```python
from build123d import *

# Parameters (mm, degrees)
ESQUISSE1_W             = 30
ESQUISSE1_H             = 30
BOSS_EXTRU_1_DEPTH      = 11
TROU_TARAUD_M31_D       = 2.5
ENL_V_MAT_EXTRU_1_REACH = 25.896
ESQUISSE6_R             = 10.5
BOSS_EXTRU_2_DEPTH      = 3.5
ESQUISSE7_R             = 8.75
BOSS_EXTRU_3_DEPTH      = 0.5
ESQUISSE8_R             = 2.5
BOSS_EXTRU_4_DEPTH      = 4
ESQUISSE9_R             = 2
BOSS_EXTRU_5_DEPTH      = 20
CHANFREIN1_SIZE         = 3
ENL_V_MAT_EXTRU_2_DEPTH = 3


with BuildPart() as part:
    # Esquisse1 → Boss.-Extru.1 (new body)
    with BuildSketch(Plane.XY):
        Rectangle(ESQUISSE1_W, ESQUISSE1_H)
    extrude(amount=BOSS_EXTRU_1_DEPTH)

    # Trou taraudé M31 (through all)
    with Locations(Plane.XY.offset(11)):
        with Locations((11, -11), (-11, 11)):
            Hole(TROU_TARAUD_M31_D / 2)

    # Esquisse5 → Enlèv. mat.-Extru.1 (cut, up to next)
    with BuildSketch(Plane.XY.offset(11), mode=Mode.PRIVATE) as enl_v_mat_extru_1_sk1:
        with BuildLine():
            Line((12.5, 12.5), (7.5, 12.5))
            ThreePointArc((7.5, 12.5), (6, 11), (7.5, 9.5))
            Line((7.5, 9.5), (12.5, 9.5))
            ThreePointArc((12.5, 9.5), (14, 11), (12.5, 12.5))
        make_face()
    enl_v_mat_extru_1_tool1 = extrude(enl_v_mat_extru_1_sk1.sketch, amount=-ENL_V_MAT_EXTRU_1_REACH, mode=Mode.PRIVATE) & part.part
    # Esquisse5 → Enlèv. mat.-Extru.1 (cut, up to next)
    with BuildSketch(Plane.XY.offset(11), mode=Mode.PRIVATE) as enl_v_mat_extru_1_sk2:
        with BuildLine():
            Line((-7.5, -9.5), (-12.5, -9.5))
            ThreePointArc((-12.5, -9.5), (-14, -11), (-12.5, -12.5))
            Line((-12.5, -12.5), (-7.5, -12.5))
            ThreePointArc((-7.5, -12.5), (-6, -11), (-7.5, -9.5))
        make_face()
    enl_v_mat_extru_1_tool2 = extrude(enl_v_mat_extru_1_sk2.sketch, amount=-ENL_V_MAT_EXTRU_1_REACH, mode=Mode.PRIVATE) & part.part
    add(enl_v_mat_extru_1_tool1.solids().sort_by_distance((10, 11, 11))[0], mode=Mode.SUBTRACT)
    add(enl_v_mat_extru_1_tool2.solids().sort_by_distance((-10, -11, 11))[0], mode=Mode.SUBTRACT)

    # Esquisse6 → Boss.-Extru.2 (add)
    with BuildSketch(Plane.XY.offset(11)):
        Circle(ESQUISSE6_R)
    extrude(amount=BOSS_EXTRU_2_DEPTH)

    # Esquisse7 → Boss.-Extru.3 (add)
    with BuildSketch(Plane.XY.offset(14.5)):
        Circle(ESQUISSE7_R)
    extrude(amount=BOSS_EXTRU_3_DEPTH)

    # Esquisse8 → Boss.-Extru.4 (add)
    with BuildSketch(Plane(origin=(0, -15, 0), x_dir=(-1, 0, 0), z_dir=(0, -1, 0))):
        with Locations(Location((0, -5.5, 0), (0, 0, 270))):
            Circle(ESQUISSE8_R)
    extrude(amount=BOSS_EXTRU_4_DEPTH)

    # Esquisse9 → Boss.-Extru.5 (add)
    with BuildSketch(Plane(origin=(0, -19, 0), x_dir=(-1, 0, 0), z_dir=(0, -1, 0))):
        with Locations(Location((0, -5.5, 0), (0, 0, 90))):
            Circle(ESQUISSE9_R)
    extrude(amount=BOSS_EXTRU_5_DEPTH)

    # Chanfrein1
    chanfrein1_edges = [part.edges().sort_by_distance(p)[0] for p in [
        (-15, 15, 5.5),
        (15, 15, 5.5),
        (15, -15, 5.5),
        (-15, -15, 5.5),
    ]]
    chamfer(chanfrein1_edges, length=CHANFREIN1_SIZE)

    # Esquisse10 → Enlèv. mat.-Extru.2 (cut)
    with BuildSketch(Plane(origin=(0, 0, 0), x_dir=(-1, 0, 0), z_dir=(0, 0, -1))):
        with BuildLine():
            Line((-7.5, 8), (-12.5, 8))
            Line((-12.5, 8), (-12.5, -7.964466094))
            Line((-12.5, -7.964466094), (-10.964466094, -7.964466094))
            ThreePointArc((-10.964466094, -7.964466094), (-8.843145751, -8.843145751), (-7.964466094, -10.964466094))
            Line((-7.964466094, -10.964466094), (-7.964466094, -12.5))
            Line((-7.964466094, -12.5), (4.5, -12.5))
            Line((4.5, -12.5), (4.5, -11))
            ThreePointArc((4.5, -11), (5.378679656, -8.878679656), (7.5, -8))
            Line((7.5, -8), (12.5, -8))
            Line((12.5, -8), (12.5, 8))
            Line((12.5, 8), (11, 8))
            ThreePointArc((11, 8), (8.878679656, 8.878679656), (8, 11))
            Line((8, 11), (8, 12.5))
            Line((8, 12.5), (-4.5, 12.5))
            Line((-4.5, 12.5), (-4.5, 11))
            ThreePointArc((-4.5, 11), (-5.378679656, 8.878679656), (-7.5, 8))
        make_face()
    extrude(amount=-ENL_V_MAT_EXTRU_2_DEPTH, mode=Mode.SUBTRACT)


solid = part.part
```
The listing builds one solid part. Answer for the finished solid, in the listing's coordinates (mm). A direction names the side the tool comes from. Give positions to 0.01 mm unless a question says otherwise; leave off trailing zeros. Order: outer loops, then holes, each group sorted by start corner. A loop starts at its lowest first (then second) coordinate and runs counter-clockwise, first axis right, second up. Notation, with made-up numbers: (46, -38.75) - (51, -38.75) arc R14 cw to (51, -31.75) - close; hole circle Ø11 at (-13.5, 71.5). An arc over 180 degrees is marked (long way). Use one line per item in the form item = value. Start each with the question number.
(1) A cutting plane is placed at D-D, the plane z = 5.5. Write down the section's boundary in (x, y).
(2) A cutting plane is placed at B-B, the plane y = 0. Write down the section's boundary in (x, z).
(3) A cutting plane is placed at C-C, the plane x = 0. Write down the section's boundary in (y, z).
(4) Consider line 1 (Y direction, x = -11, z = 7); line 2 (Y direction, x = 11, z = 7.5); line 3 (Y direction, x = 8.5, z = 10). Determine where each line is inside the solid, lowest interval first. Write a range as from..to.
(5) Flat-ended cylindrical pins translate along their axes: pin 1 Ø1 at (x, y) = (3, -1.5) entering from -Z; pin 2 Ø2.5 at (x, z) = (10, 1) entering from -Y; pin 3 Ø6 at (y, z) = (-28.5, 8.5) entering from +X. Find the tip coordinate at first contact, or state that the pin passes through.
(6) A cutting plane is placed at A-A, the plane z = 9.75. Write down the section's boundary in (x, y), then the cut area to 3 significant figures.
(7) The mould has two halves that part along X. Classify faces 1 (the flat face through (-15, 0, 5)), 2 (the flat face through (-4, 8, 14.5)), 3 (the flat face through (-10, -12.5, 6)), 4 (the cylindrical face through (11.921, -10.155, 5.423)): released by +X, released by -X, zero draft, split by the parting line, or undercut.
(8) For faces 5 (the cylindrical face through (-14, -11, 6)), 6 (the cylindrical face through (10, 3.2, 12.7)), 7 (the flat face through (-12.5, 0, 1)), determine the directions among +Z, -Z, +X, -X, +Y, -Y from which every point of the face is accessible in a straight line to the end or side of a thin tool.
Ans:
q1.outline = (-15, -12) - (-12, -15) - (-2.5, -15) - (-2.5, -19) - (-2, -19) - (-2, -39) - (2, -39) - (2, -19) - (2.5, -19) - (2.5, -15) - (12, -15) - (15, -12) - (15, 12) - (12, 15) - (-12, 15) - (-15, 12) - close; hole (-12.5, -12.5) - (-7.5, -12.5) arc R1.5 ccw to (-7.5, -9.5) - (-12.5, -9.5) arc R1.5 ccw to start; hole circle Ø2.5 at (-11, 11); hole (7.5, 9.5) - (12.5, 9.5) arc R1.5 ccw to (12.5, 12.5) - (7.5, 12.5) arc R1.5 ccw to start; hole circle Ø2.5 at (11, -11)
q2.outline = (-15, 0) - (-12.5, 0) - (-12.5, 3) - (12.5, 3) - (12.5, 0) - (15, 0) - (15, 11) - (10.5, 11) - (10.5, 14.5) - (8.75, 14.5) - (8.75, 15) - (-8.75, 15) - (-8.75, 14.5) - (-10.5, 14.5) - (-10.5, 11) - (-15, 11) - close
q3.outline = (-39, 3.5) - (-19, 3.5) - (-19, 3) - (-15, 3) - (-15, 0) - (-12.5, 0) - (-12.5, 3) - (12.5, 3) - (12.5, 0) - (15, 0) - (15, 11) - (10.5, 11) - (10.5, 14.5) - (8.75, 14.5) - (8.75, 15) - (-8.75, 15) - (-8.75, 14.5) - (-10.5, 14.5) - (-10.5, 11) - (-15, 11) - (-15, 8) - (-19, 8) - (-19, 7.5) - (-39, 7.5) - close
q4.line_1 = -15..-12.5, -9.5..9.75, 12.25..15
q4.line_2 = -15..-12.25, -9.75..9.5, 12.5..15
q4.line_3 = -15..9.5, 12.5..15
q5.pin_1 = 3
q5.pin_2 = -15
q5.pin_3 = 2
q6.outline = (-15, -12) - (-12, -15) - (12, -15) - (15, -12) - (15, 12) - (12, 15) - (-12, 15) - (-15, 12) - close; hole (-12.5, -12.5) - (-7.5, -12.5) arc R1.5 ccw to (-7.5, -9.5) - (-12.5, -9.5) arc R1.5 ccw to start; hole circle Ø2.5 at (-11, 11); hole (7.5, 9.5) - (12.5, 9.5) arc R1.5 ccw to (12.5, 12.5) - (7.5, 12.5) arc R1.5 ccw to start; hole circle Ø2.5 at (11, -11)
q6.area = 828 mm^2
q7.face_1 = released by -X
q7.face_2 = zero draft
q7.face_3 = undercut
q7.face_4 = undercut
q8.face_5 = +Z, -Z
q8.face_6 = +Z
q8.face_7 = -Z
